CAD build for the part. Positions are in the model's coordinates, mm. A direction names the side the tool comes from. Round coordinates to 2 decimals unless told otherwise and drop trailing zeros. Write each loop counter-clockwise with the first axis right and the second up, starting at its lowest first coordinate (ties: lowest second). Pieces come first, ordered by that corner, then holes. Notation, with made-up numbers: (32, -8.5) - (87, -8.5) arc R11 ccw to (87, 12.5) - close; hole circle Ø1 at (-18.5, -2.75). An arc over 180 degrees is marked (long way). Answer in a Markdown table with one row per item.
```python
from build123d import *

# Parameters (mm, degrees)
F0_W     = 200
F0_H     = 15.5
F1_DEPTH = 300
F2_W     = 13
F2_H     = 120
F3_DEPTH = 15.501
F5_W     = 10
F5_H     = 7
F6_DEPTH = 28.5


with BuildPart() as f1:
    # F0 (on Front) → F1 (new body)
    with BuildSketch(Plane.XZ):
        with Locations((100, 7.75)):
            Rectangle(F0_W, F0_H)
    extrude(amount=-F1_DEPTH)

    # F2 (on face) → F3 (cut, through all)
    with BuildSketch(Plane.XY.offset(15.5)):
        with Locations((6.5, 210)):
            Rectangle(F2_W, F2_H)
        with Locations((6.5, 90)):
            Rectangle(F2_W, F2_H)
    extrude(amount=-F3_DEPTH, mode=Mode.SUBTRACT)

    # F5 (on offset) → F6 (cut, through all)
    with BuildSketch(Plane.XZ.offset(-1.5)):
        with Locations((6.5, 10.4964849353)):
            Rectangle(F5_W, F5_H)
    extrude(amount=-F6_DEPTH, mode=Mode.SUBTRACT)


solid = f1.part
```
Q1. Flat gauge pin, fed straight in: pin 1 (2 mm diameter, centred on y = 202.5, z = 10, fed in from -X). Where does the tip first touch, or does it go through?
Computed:
| item | result |
|---|---|
| pin 1 | stops at x = 13 |
Q2. Saw through at B-B on y = 83. List the corners of the cut face in (x, z), then the cut area to 3 significant figures.
Computed:
| item | result |
|---|---|
| outline | (13, 0) - (200, 0) - (200, 15.5) - (13, 15.5) - close |
| area | 2,900 mm2 |
Q3. Drill centre lines: line 1 (X direction, y = 87.5, z = 13.5); line 2 (X direction, y = 23.5, z = 10.75). Where is each one in solid material? Low to high.
Computed:
| item | result |
|---|---|
| line 1 | x = 13 to 200 |
| line 2 | x = 0 to 1.5, 11.5 to 200 |
Q4. 3-axis set-ups, long thin cutter, end or side, ignore diameter. For faces 5 (the flat face through (200, 148, 8)), 6 (the flat face through (6, 270, 8)), 7 (the flat face through (6, 1.5, 11)): which of +Z, -Z, +X, -X, +Y, -Y reach the whole face in a straight line?
Computed:
| item | result |
|---|---|
| face 5 | +Z, -Z, +X, +Y, -Y |
| face 6 | +Z, -Z, -X |
| face 7 | none |
Q5. Saw through at A-A on z = 10.75. List the corners of the cut face in (x, y).
Computed:
| item | result |
|---|---|
| outline | (0, 0) - (200, 0) - (200, 300) - (0, 300) - (0, 270) - (13, 270) - (13, 30) - (11.5, 30) - (11.5, 1.5) - (1.5, 1.5) - (1.5, 30) - (0, 30) - close |
Q6. Pull direction Y, two halves, no side cores. Call faces 1 (the flat face through (6, 16, 13.996)), 2 (the flat face through (99, 0, 8)), 3 (the flat face through (0, 15, 8)), 4 (the flat face through (99, 300, 8)): released by +Y, released by -Y, zero draft, split by the parting line, or undercut.
Computed:
| item | result |
|---|---|
| face 1 | undercut |
| face 2 | released by -Y |
| face 3 | zero draft |
| face 4 | released by +Y |
